```python
from build123d import *
from build123d import SkipClean  # not in build123d's __all__

# Parameters (mm, degrees)
F4_D     = 12.7
F5_R     = 128.2794587314
F5_R_2   = 6.35
F5_R_3   = 60.7691295445
F6_DEPTH = 25.4


with BuildPart() as f2:
    # F0 (on Front) → F2 (revolve)
    with BuildSketch(Plane.XZ):
        Polygon((-52.4943843484, 27.3255631328), (-32.0674665272, 27.3255631328), (-32.0674665272, 113.4814321995), (-32.0674665272, 146.3606357574), (-53.1988926232, 146.3606357574), (-53.1988926232, 122.2296878695), (-116.6306659579, 122.2296878695), (-114.9781197309, 147.7223485708), (-146.413102746, 147.7223485708), (-146.413102746, 94.8358923197), (-52.4943843484, 94.8358923197), align=None)
    revolve(axis=Axis((-79.9387739971, 0, -33.4435664117), (1, 0, 0)))

    # F4 (through all)
    with Locations(Plane(origin=(-52.4943843484, 0, 0), x_dir=(0, -1, 0), z_dir=(-1, 0, 0))):
        with Locations((-68.8715130091, -89.2082676291)):
            Hole(F4_D / 2)

    # F5 (on face) → F6 (join)
    with BuildSketch(Plane(origin=(-52.4943843484, 0, 0), x_dir=(0, -1, 0), z_dir=(-1, 0, 0))):
        with Locations((0, -33.4435664117)):
            Circle(F5_R)
        with Locations((-68.8715130091, -89.2082676291)):
            Circle(F5_R_2, mode=Mode.SUBTRACT)
        with Locations((0, -33.4435664117)):
            Circle(F5_R_3, mode=Mode.SUBTRACT)
    with SkipClean():  # cleaning this boolean's faces spoils the solid; the shape is the same uncleaned
        extrude(amount=F6_DEPTH)


solid = f2.part
```
The listing builds one solid part. Answer for the finished solid, in the listing's coordinates (mm). A direction names the side the tool comes from. Coordinates: 2 decimals unless noted, no trailing zeros. Loops run counter-clockwise (first coordinate to the right, second up) from the corner with the lowest first, then second, coordinate; pieces in that order, holes last. Notation, with made-up numbers: (20, 74) -> (30, 74) arc R9 cw to (30, 89) -> close; hole circle Ø9 at (66.5, 52.25). An arc over 180 degrees is marked (long way). Return JSON: item names as keys, results as strings. Group by question number.
(1) Find the intervals of material crossed by probe 1 along Z at (x, y) = (-38, 0); probe 2 along Z at (x, y) = (-57, 0); probe 3 along X at (y, z) = (-15, 27.5), in increasing order. Write a range as from..to.
(2) Given pin 1 Ø5 at (x, z) = (-101, -117) entering from -Y; pin 2 Ø16.5 at (y, z) = (68.87, -89.21) entering from -X; pin 3 Ø8 at (x, y) = (-70, -9) entering from -Z, each flat-ended and moving along its own axis, determine where each tip first touches the part or whether it passes through.
(3) Determine the mould class of faces 4 (the flat face through (-77.894, -55, -60)), 5 (the flat face through (-146.413, 38, -157)), 6 (the cylindrical face through (-42.78, 175.53, -72.42)) for opening direction Y: released by +Y, released by -Y, zero draft, split by the parting line, or undercut.
(4) A cutting plane is placed at A-A on y = 0. Write down the section's boundary in (x, z), and give its area (3 significant figures).
(5) Which of the six approach directions +Z, -Z, +X, -X, +Y, -Y give full straight-line access (tool end or side, diameter ignored) to faces 1 (the cylindrical face through (-130.916, -54.417, 139.356)), 2 (the cylindrical face through (-111.674, 113.806, 25.75)), 3 (the cylindrical face through (-85.36, -46.76, 115.04))?
The answers:
{
 "1": {"probe 1": "z = -213.25..-94.21, 27.33..146.36", "probe 2": "z = -189.12..-94.21, 27.33..122.23", "probe 3": "x = -77.89..-32.07"},
 "2": {"pin 1": "stops at y = -132.91", "pin 2": "stops at x = -77.89", "pin 3": "stops at z = -189.04"},
 "3": {"face 4": "undercut", "face 5": "zero draft", "face 6": "split by the parting line"},
 "4": {"outline": "(-146.41, -214.61) -> (-114.98, -214.61) -> (-116.63, -189.12) -> (-53.2, -189.12) -> (-53.2, -213.25) -> (-32.07, -213.25) -> (-32.07, -94.21) -> (-77.89, -94.21) -> (-77.89, -161.72) -> (-146.41, -161.72) -> close; (-146.41, 94.84) -> (-77.89, 94.84) -> (-77.89, 27.33) -> (-32.07, 27.33) -> (-32.07, 146.36) -> (-53.2, 146.36) -> (-53.2, 122.23) -> (-116.63, 122.23) -> (-114.98, 147.72) -> (-146.41, 147.72) -> close", "area": "15,000 mm^2"},
 "5": {"face 1": "+X, -X", "face 2": "-X", "face 3": "none"}
}
